Model file for the job. Use its own axes, mm. Face numbers are marked on the shaded views. A direction names the side the tool comes from. Round coordinates to 2 decimals unless told otherwise and drop trailing zeros. Order: outer loops, then holes, each group sorted by start corner. A loop starts at its lowest first (then second) coordinate and runs counter-clockwise, first axis right, second up. Notation, with made-up numbers: (79, -3) -> (98, -3) arc R18 cw to (98, 11) -> close; hole circle Ø8 at (28.5, -16). An arc over 180 degrees is marked (long way). Put each result on its own line as item: value. Start each with the question number.
Q1. Cut at A-A, the plane y = 46. List the corners of the cut face in (x, z), and give its area (3 significant figures).
Q2. Flat gauge pins, fed straight in: P1, Ø3.5, axis at x = -26.5, z = -6.99, coming from the +Y side; P2, Ø5, axis at y = 46, z = 3, coming from the +X side; P3, Ø1.2, axis at x = -10, z = 0, coming from the +Y side; P4, Ø2.5, axis at x = -5.5, z = 7, coming from the +Y side. Where does each tip first touch, or does it go through?
Q3. Cut at B-B, the plane z = 3. State how many separate pieces and enclosed holes the cut face has, and give its area (3 significant figures).
Q4. Probe L1, parallel to Z at x = -19.5, y = 53.5; L2, parallel to X at y = 50.5, z = 0; L3, parallel to X at y = 37, z = -0.5. List the from-to ranges inside material, lowest first.
Q5. Pull direction Z, two halves, no side cores. Call the marked faces 1, 2 and 3: released by +Z, released by -Z, zero draft, split by the parting line, or undercut.
Q6. 3-axis set-ups, long thin cutter, end or side, ignore diameter. For the marked faces 4 and 5: which of +Z, -Z, +X, -X, +Y, -Y reach the whole face in a straight line?
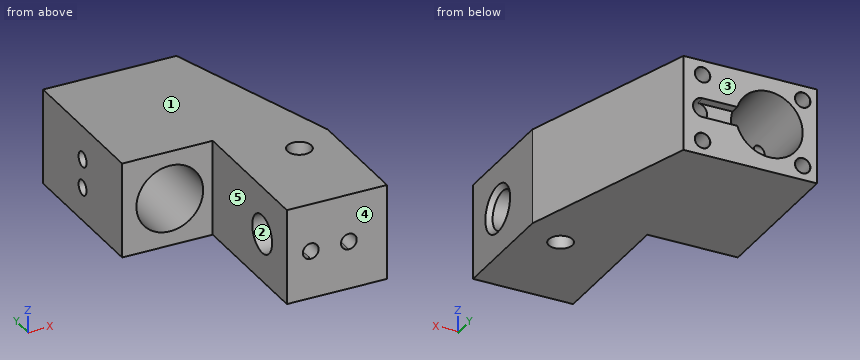
from build123d import *

# Parameters (mm, degrees)
SKETCH1_W                      = 21
SKETCH1_H                      = 20
BOSS_EXTRUDE2_DEPTH            = 62
CUT_EXTRUDE1_DEPTH             = 62
SKETCH4_W                      = 20
SKETCH4_H                      = 32
BOSS_EXTRUDE3_DEPTH            = 19
SKETCH7_R                      = 7
CUT_EXTRUDE2_DEPTH             = 47
SKETCH8_R                      = 4
CUT_EXTRUDE3_DEPTH             = 47
M3_CLEARANCE_HOLE1_D           = 3.2
M3_CLEARANCE_HOLE1_DEPTH       = 22.15862301
M3_CLEARANCE_HOLE1_CSINK_D     = 3.25
M3_CLEARANCE_HOLE1_CSINK_ANGLE = 90
M3_CLEARANCE_HOLE1_TIP         = 0.96137699
CUT_EXTRUDE7_DEPTH             = 72.513984646
CUT_EXTRUDE7_DEPTH_BACK        = 72.513984646
SKETCH14_R                     = 2.5
CHAMFER1_SIZE                  = 1
CUT_EXTRUDE8_DEPTH             = 2
HOLE1_D                        = 2.5
HOLE1_DEPTH                    = 100
SKETCH18_R                     = 2
CUT_EXTRUDE10_DEPTH            = 30
SKETCH19_R                     = 1.6
CUT_EXTRUDE11_DEPTH            = 13
CUT_EXTRUDE12_REACH            = 71.385
CUT_EXTRUDE12_END_RADIUS       = 2.5
SKETCH24_R                     = 1.65


with BuildPart() as part:
    # Sketch1 → Boss-Extrude2 (new body)
    with BuildSketch(Plane(origin=(0, 0, 0), x_dir=(1, 0, 0), z_dir=(0, 1, 0))):
        Rectangle(SKETCH1_W, SKETCH1_H)
    extrude(amount=BOSS_EXTRUDE2_DEPTH)

    # Sketch3 → Cut-Extrude1 (cut)
    with BuildSketch(Plane.XY.offset(10)):
        Polygon((10.5, 62), (-1.5, 62), (10.5, 24), align=None)
    extrude(amount=-CUT_EXTRUDE1_DEPTH, mode=Mode.SUBTRACT)

    # Sketch4 → Boss-Extrude3 (add)
    with BuildSketch(Plane.ZY.offset(10.5)):
        with Locations((0, 46)):
            Rectangle(SKETCH4_W, SKETCH4_H)
    extrude(amount=BOSS_EXTRUDE3_DEPTH)

    # Sketch7 → Cut-Extrude2 (cut)
    with BuildSketch(Plane(origin=(0, 62, 0), x_dir=(1, 0, 0), z_dir=(0, 1, 0))):
        with Locations(Location((-19.5, 0, 0), (0, 0, 270))):
            Circle(SKETCH7_R)
    extrude(amount=-CUT_EXTRUDE2_DEPTH, mode=Mode.SUBTRACT)

    # Sketch8 → Cut-Extrude3 (cut)
    with BuildSketch(Plane(origin=(10.5, 0, 0), x_dir=(0, 0, -1), z_dir=(1, 0, 0))):
        with Locations((0, 10)):
            Circle(SKETCH8_R)
    extrude(amount=-CUT_EXTRUDE3_DEPTH, mode=Mode.SUBTRACT)

    # M3 Clearance Hole1
    with Locations(Plane(origin=(0, 62, 0), x_dir=(1, 0, 0), z_dir=(0, 1, 0))):
        with Locations((-26.5, 6.988952109), (-26.5, -6.988952109), (-5.5, -7), (-5.5, 7)):
            CounterSinkHole(M3_CLEARANCE_HOLE1_D / 2, M3_CLEARANCE_HOLE1_CSINK_D / 2, depth=M3_CLEARANCE_HOLE1_DEPTH, counter_sink_angle=M3_CLEARANCE_HOLE1_CSINK_ANGLE)
            with Locations((0, 0, -(M3_CLEARANCE_HOLE1_DEPTH + M3_CLEARANCE_HOLE1_TIP / 2))):  # 118° drill point
                Cone(0, M3_CLEARANCE_HOLE1_D / 2, M3_CLEARANCE_HOLE1_TIP, mode=Mode.SUBTRACT)

    # Sketch14 → Cut-Extrude7 (cut, two sides: drawn at the far end of the back side and taken through both)
    with BuildSketch(Plane.XY.offset(10).offset(-CUT_EXTRUDE7_DEPTH_BACK)):
        with Locations((2.5, 20)):
            Circle(SKETCH14_R)
    extrude(amount=CUT_EXTRUDE7_DEPTH + CUT_EXTRUDE7_DEPTH_BACK, mode=Mode.SUBTRACT)

    # Chamfer1
    chamfer1_edges = [part.edges().sort_by_distance(p)[0] for p in [
        (10.5, 10, 4),
    ]]
    chamfer(chamfer1_edges, length=CHAMFER1_SIZE)

    # Sketch15 → Cut-Extrude8 (cut)
    with BuildSketch(Plane(origin=(0, 62, 0), x_dir=(1, 0, 0), z_dir=(0, 1, 0))):
        with BuildLine():
            Line((-5.5, 2), (-14.947436463, 2))
            Line((-14.947436463, 2), (-14.947436463, -2))
            Line((-14.947436463, -2), (-5.5, -2))
            ThreePointArc((-5.5, -2), (-3.5, 0), (-5.5, 2))
        make_face()
    extrude(amount=-CUT_EXTRUDE8_DEPTH, mode=Mode.SUBTRACT)

    # Hole1
    with Locations(Plane(origin=(0, 60, 0), x_dir=(1, 0, 0), z_dir=(0, 1, 0))):
        with Locations((-5.231662338, 0)):
            Hole(HOLE1_D / 2, depth=HOLE1_DEPTH)

    # Sketch18 → Cut-Extrude10 (cut)
    with BuildSketch(Plane(origin=(0, 60, 0), x_dir=(1, 0, 0), z_dir=(0, 1, 0))):
        with Locations(Location((-5.5, 0, 0), (0, 0, 270))):
            Circle(SKETCH18_R)
    extrude(amount=-CUT_EXTRUDE10_DEPTH, mode=Mode.SUBTRACT)

    # Sketch19 → Cut-Extrude11 (cut)
    with BuildSketch(Plane.ZY.offset(29.5)):
        with Locations((-3, 46)):
            Circle(SKETCH19_R)
        with Locations((3, 46)):
            Circle(SKETCH19_R)
    extrude(amount=-CUT_EXTRUDE11_DEPTH, mode=Mode.SUBTRACT)

    # M4 Tapped Hole1: read off the stored shape, not the designer's step
    # M4 Tapped Hole1: loft between two sections, ruled curve by curve
    m4_tapped_hole1_from = [
        Edge.make_three_point_arc((-5.5, 6.356330866, -1.65), (-3.85, 6.356330866, 0), (-5.5, 6.356330866, 1.65)),
        Edge.make_three_point_arc((-5.5, 6.356330866, 1.65), (-7.15, 6.356330866, 0), (-5.5, 6.356330866, -1.65)),
    ]
    m4_tapped_hole1_to = [
        Edge.make_three_point_arc((-5.5, 0, -1.65), (-3.85, 0, 0), (-5.5, 0, 1.65)),
        Edge.make_three_point_arc((-5.5, 0, 1.65), (-7.15, 0, 0), (-5.5, 0, -1.65)),
    ]
    m4_tapped_hole1 = Solid(Shell([*[Face.make_surface_from_curves(m4_tapped_hole1_from[k], m4_tapped_hole1_to[k]) for k in range(2)], Face(Wire(m4_tapped_hole1_from)), Face(Wire(m4_tapped_hole1_to))]))
    add(m4_tapped_hole1, mode=Mode.SUBTRACT)

    # M4 Tapped Hole1 2: loft between two sections, ruled curve by curve
    m4_tapped_hole1_2_from = [
        Edge.make_three_point_arc((-5.5, 30, -1.65), (-3.85, 30, 0), (-5.5, 30, 1.65)),
        Edge.make_three_point_arc((-5.5, 30, 1.65), (-7.15, 30, 0), (-5.5, 30, -1.65)),
    ]
    m4_tapped_hole1_2_to = [
        Edge.make_three_point_arc((-5.5, 13.643669134, -1.65), (-3.85, 13.643669134, 0), (-5.5, 13.643669134, 1.65)),
        Edge.make_three_point_arc((-5.5, 13.643669134, 1.65), (-7.15, 13.643669134, 0), (-5.5, 13.643669134, -1.65)),
    ]
    m4_tapped_hole1_2 = Solid(Shell([*[Face.make_surface_from_curves(m4_tapped_hole1_2_from[k], m4_tapped_hole1_2_to[k]) for k in range(2)], Face(Wire(m4_tapped_hole1_2_from)), Face(Wire(m4_tapped_hole1_2_to))]))
    add(m4_tapped_hole1_2, mode=Mode.SUBTRACT)

    # M4 Tapped Hole1 3: loft between two sections, ruled curve by curve
    m4_tapped_hole1_3_from = [
        Edge.make_three_point_arc((2.5, 6.356330866, -1.65), (4.15, 6.356330866, 0), (2.5, 6.356330866, 1.65)),
        Edge.make_three_point_arc((2.5, 6.356330866, 1.65), (0.85, 6.356330866, 0), (2.5, 6.356330866, -1.65)),
    ]
    m4_tapped_hole1_3_to = [
        Edge.make_three_point_arc((2.5, 0, -1.65), (4.15, 0, 0), (2.5, 0, 1.65)),
        Edge.make_three_point_arc((2.5, 0, 1.65), (0.85, 0, 0), (2.5, 0, -1.65)),
    ]
    m4_tapped_hole1_3 = Solid(Shell([*[Face.make_surface_from_curves(m4_tapped_hole1_3_from[k], m4_tapped_hole1_3_to[k]) for k in range(2)], Face(Wire(m4_tapped_hole1_3_from)), Face(Wire(m4_tapped_hole1_3_to))]))
    add(m4_tapped_hole1_3, mode=Mode.SUBTRACT)

    # Cut-Extrude12: up to this cylinder (the profile starts outside it)
    cut_extrude12_end = Plane(origin=(2.5, 20, 0), z_dir=(0, 0, 1)) * Cylinder(CUT_EXTRUDE12_END_RADIUS, 148.77, mode=Mode.PRIVATE)
    # Sketch24 → Cut-Extrude12 (cut, up to the surface)
    with BuildSketch(Plane.XZ, mode=Mode.PRIVATE) as cut_extrude12_sk1:
        with Locations(Location((2.5, 0, 0), (0, 0, 270))):
            Circle(SKETCH24_R)
    cut_extrude12_tool1 = extrude(cut_extrude12_sk1.sketch, amount=-CUT_EXTRUDE12_REACH, mode=Mode.PRIVATE) - cut_extrude12_end
    add(cut_extrude12_tool1.solids().sort_by_distance((2.5, 0, 0))[0], mode=Mode.SUBTRACT)


solid = part.part
Ans:
1. outline: (-29.5, -10) -> (3.55, -10) -> (3.55, 10) -> (-29.5, 10) -> (-29.5, 4.6) -> (-24.78, 4.6) arc R7 cw (long way) to (-24.78, -4.6) -> (-29.5, -4.6) -> close; (-29.5, -1.4) -> (-26.36, -1.4) arc R7 cw to (-26.36, 1.4) -> (-29.5, 1.4) -> close; hole circle Ø3.2 at (-26.5, -6.99); hole circle Ø3.2 at (-26.5, 6.99); hole circle Ø4 at (-5.5, 0); hole circle Ø3.2 at (-5.5, -7); hole circle Ø3.2 at (-5.5, 7)
1. area: 438 mm^2
2. P1: stops at y = 62
2. P2: stops at x = 4.34
2. P3: stops at y = 60
2. P4: stops at y = 39.63
3. separate pieces: 4
3. enclosed holes: 1
3. area: 1,130 mm^2
4. L1: z = -10 to -7, 7 to 10
4. L2: x = -29.5 to -26.5, -12.5 to -7.5, -3.5 to 2.13
4. L3: x = -29.5 to -26.48, -12.52 to -7.44, -3.56 to 6.39
5. face 1: released by +Z
5. face 2: undercut
5. face 3: zero draft
6. face 4: +Z, -Z, +X, -X, -Y
6. face 5: +Z, -Z, -X, -Y
